```python
from build123d import *

# Parameters (mm, degrees)
F0_W           = 55
F0_H           = 45
F1_DEPTH       = 15
F3_D           = 12.5
F3_DEPTH       = 15
F4_D           = 6
F4_DEPTH       = 15
F4_CSINK_D     = 10.4
F4_CSINK_ANGLE = 90


with BuildPart() as f1:
    # F0 (on Right) → F1 (new body)
    with BuildSketch(Plane.YZ):
        Rectangle(F0_W, F0_H)
    extrude(amount=F1_DEPTH)

    # F3
    with Locations(Plane.YZ.offset(15)):
        with Locations((0, 13.5)):
            Hole(F3_D / 2, depth=F3_DEPTH)

    # F4
    with Locations(Plane.YZ.offset(15)):
        with Locations((-19.5, -14.5), (0, -14.5), (19.5, -14.5)):
            CounterSinkHole(F4_D / 2, F4_CSINK_D / 2, depth=F4_DEPTH, counter_sink_angle=F4_CSINK_ANGLE)


solid = f1.part
```
Check sheet for the modelled part. Datum: model origin and axes. Units: mm. Round coordinates to 2 decimals unless told otherwise and drop trailing zeros. Order: outer loops, then holes, each group sorted by start corner. A loop starts at its lowest first (then second) coordinate and runs counter-clockwise, first axis right, second up.
1) Section check D-D (z = -14.5). Record the boundary of the cut face in (x, y), and give its area (3 significant figures).
2) Section check B-B (x = 13.75). Record the boundary of the cut face in (y, z).
3) Scan lines: line 1 (Z direction, x = 8.5, y = 0); line 2 (Y direction, x = 9.25, z = -14.5); line 3 (Z direction, x = 7.75, y = 19.5). Record each from-to range of solid material in increasing order.
4) Section check A-A (z = 13.5). Record the boundary of the cut face in (x, y), and give its area (4 significant figures).
5) Go/stop test with flat-tipped pins: pin 1 Ø5.5 at (y, z) = (-19.5, -14.5) entering from +X; pin 2 Ø9.5 at (y, z) = (0, -14.5) entering from +X. Record where each tip stops, or that it passes through.
6) Section check C-C (y = -19.5). Record the boundary of the cut face in (x, z), and give its area (3 significant figures).
7) Mould release check, pull along Y, two halves, no side actions. Record for faces 1 (the cylindrical face through (6.31, -18.85, -17.43)), 2 (the flat face through (7, 0, -22.5)), 3 (the flat face through (7, -27.5, 0)): +Y half, -Y half, draft (parallel to the pull), parting line (faces both ways), or undercut.
Result:
1. outline: (0, -27.5) - (15, -27.5) - (15, -24.7) - (12.8, -22.5) - (0, -22.5) - close; (0, -16.5) - (12.8, -16.5) - (15, -14.3) - (15, -5.2) - (12.8, -3) - (0, -3) - close; (0, 3) - (12.8, 3) - (15, 5.2) - (15, 14.3) - (12.8, 16.5) - (0, 16.5) - close; (0, 22.5) - (12.8, 22.5) - (15, 24.7) - (15, 27.5) - (0, 27.5) - close
1. area: 540 mm2
2. outline: (-27.5, -22.5) - (27.5, -22.5) - (27.5, 22.5) - (-27.5, 22.5) - close; hole circle Ø7.9 at (-19.5, -14.5); hole circle Ø12.5 at (0, 13.5); hole circle Ø7.9 at (0, -14.5); hole circle Ø7.9 at (19.5, -14.5)
3. line 1: z = -22.5 to -17.5, -11.5 to 7.25, 19.75 to 22.5
3. line 2: y = -27.5 to -22.5, -16.5 to -3, 3 to 16.5, 22.5 to 27.5
3. line 3: z = -22.5 to -17.5, -11.5 to 22.5
4. outline: (0, -27.5) - (15, -27.5) - (15, -6.25) - (0, -6.25) - close; (0, 6.25) - (15, 6.25) - (15, 27.5) - (0, 27.5) - close
4. area: 637.5 mm2
5. pin 1: passes through
5. pin 2: stops at x = 14.55
6. outline: (0, -22.5) - (15, -22.5) - (15, -19.7) - (12.8, -17.5) - (0, -17.5) - close; (0, -11.5) - (12.8, -11.5) - (15, -9.3) - (15, 22.5) - (0, 22.5) - close
6. area: 580 mm2
7. face 1: undercut
7. face 2: draft
7. face 3: -Y half
